from build123d import *

# Parameters (mm, degrees)
SKETCH1_R            = 15
BOSS_EXTRUDE1_DEPTH  = 2.75
SKETCH1_3_W          = 2
SKETCH1_3_H          = 25
BOSS_EXTRUDE2_DEPTH  = 4.25
CUT_EXTRUDE1_DEPTH   = 49.073511417
M4_CLEARANCE_HOLE1_D = 4.5


with BuildPart() as part:
    # Sketch1 → Boss-Extrude1 (new, symmetric)
    with BuildSketch(Plane.XY):
        Polygon((19, 12.5), (21, 12.5), (10, 23), (10, 21), (-10, 21), (-10, 23), (-21, 12.5), (-19, 12.5), (-19, -12.5), (-21, -12.5), (-21, -23), (-17, -23), (-17, -20), (-14, -20), (-14, -23), (-10, -23), (-10, -21), (10, -21), (10, -23), (14, -23), (14, -20), (17, -20), (17, -23), (21, -23), (21, -12.5), (19, -12.5), align=None)
        Circle(SKETCH1_R, mode=Mode.SUBTRACT)
    extrude(amount=BOSS_EXTRUDE1_DEPTH, both=True)

    # Sketch1<3> → Boss-Extrude2 (add, symmetric)
    with BuildSketch(Plane.XY):
        with Locations((-20, 0)):
            Rectangle(SKETCH1_3_W, SKETCH1_3_H)
        with Locations((20, 0)):
            Rectangle(SKETCH1_3_W, SKETCH1_3_H)
    extrude(amount=BOSS_EXTRUDE2_DEPTH, both=True)

    # Sketch2 → Cut-Extrude1 (cut, through all)
    with BuildSketch(Plane.ZY.offset(21)):
        Polygon((4.25, -12.5), (4.25, -8.5), (2.75, -12.5), align=None)
        Polygon((-2.75, -12.5), (-4.25, -8.5), (-4.25, -12.5), align=None)
        Polygon((-4.25, 8.5), (-2.75, 12.5), (-4.25, 12.5), align=None)
        Polygon((4.25, 12.5), (2.75, 12.5), (4.25, 8.5), align=None)
    extrude(amount=-CUT_EXTRUDE1_DEPTH, mode=Mode.SUBTRACT)

    # M4 Clearance Hole1 (through all)
    with Locations(Plane(origin=(0, 21, 0), x_dir=(1, 0, 0), z_dir=(0, 1, 0))):
        with Locations((0, 0)):
            Hole(M4_CLEARANCE_HOLE1_D / 2)


solid = part.part
Work out the finished part from the listing and answer in its coordinate system (mm). A direction names the side the tool comes from. Round coordinates to 2 decimals unless told otherwise and drop trailing zeros. Order: outer loops, then holes, each group sorted by start corner. A loop starts at its lowest first (then second) coordinate and runs counter-clockwise, first axis right, second up. Notation, with made-up numbers: M 62.25,63 L 84.25,63 A17 ccw 84.25,85 Z; hole C -31.75,-21.5 d3. An arc over 180 degrees is marked long. Put each result on its own line as item: value. Start each with the question number.
Q1. Straight lines are drawn through the part: L1, parallel to X at y = -3, z = 4; L2, parallel to Z at x = 0, y = -18.5; L3, parallel to Z at x = -6, y = 17. For each, find the intervals that lie inside material, in ascending order. Write a range as [from, to].
Q2. Section A-A, the plane x = 0 is taken. Write down the section's boundary in (y, z).
Q3. Section B-B, the plane y = 0 is taken. Write down the section's boundary in (x, z), and give its area (3 significant figures).
Q4. Section D-D, the plane x = 9 is taken. Write down the section's boundary in (y, z).
Q5. For a pull along Z with two mould halves and no side action, classify faces 1 (the flat face through (-15.423, 17.824, 0.038)), 2 (the flat face through (-5, -15, -2.75)), 3 (the cylindrical face through (0.29, -17.96, -2.23)) as pulls with the +Z half, pulls with the -Z half, needs draft (parallel to the pull), parting line crosses it, or undercut.
Q6. Flat-ended cylindrical pins translate along their axes: pin 1 (12 mm diameter, centred on x = 9, y = 1.5, fed in from +Z); pin 2 (8 mm diameter, centred on x = 14, y = 3.5, fed in from -Z); pin 3 (3.5 mm diameter, centred on x = 15, z = 0.5, fed in from -Y); pin 4 (3 mm diameter, centred on x = -2.5, z = 2.5, fed in from -Y). Find the tip coordinate at first contact, or state that the pin passes through.
Q7. Section C-C, the plane z = 0 is taken. Write down the section's boundary in (x, y).
Q8. A tool of negligible diameter and unlimited length cuts with its end or side. For faces 4 (the flat face through (10, -22, 0)), 5 (the flat face through (19, 0, -3)), 6 (the flat face through (-21, -5, 0)), 7 (the flat face through (-19, 0, 3)), 8 (the flat face through (12, -23, 0)), from which of +Z, -Z, +X, -X, +Y, -Y can it reach the whole face along a straight path? Write none if from no direction.
Findings below:
1. L1: x = [-21, -19], [19, 21]
1. L2: z = [-2.75, -2.25], [2.25, 2.75]
1. L3: z = [-2.75, 2.75]
2. outline: M -21,-2.75 L -15,-2.75 L -15,-2.25 L -21,-2.25 Z; M -21,2.25 L -15,2.25 L -15,2.75 L -21,2.75 Z; M 15,-2.75 L 21,-2.75 L 21,-2.25 L 15,-2.25 Z; M 15,2.25 L 21,2.25 L 21,2.75 L 15,2.75 Z
3. outline: M -21,-4.25 L -19,-4.25 L -19,-2.75 L -15,-2.75 L -15,2.75 L -19,2.75 L -19,4.25 L -21,4.25 Z; M 15,-2.75 L 19,-2.75 L 19,-4.25 L 21,-4.25 L 21,4.25 L 19,4.25 L 19,2.75 L 15,2.75 Z
3. area: 78.0 mm^2
4. outline: M -21,-2.75 L -12,-2.75 L -12,2.75 L -21,2.75 Z; M 12,-2.75 L 21,-2.75 L 21,2.75 L 12,2.75 Z
5. face 1: needs draft
5. face 2: pulls with the -Z half
5. face 3: undercut
6. pin 1: stops at z = 2.75
6. pin 2: stops at z = -2.75
6. pin 3: stops at y = -23
6. pin 4: stops at y = -21
7. outline: M -21,-23 L -17,-23 L -17,-20 L -14,-20 L -14,-23 L -10,-23 L -10,-21 L -2.25,-21 L -2.25,-14.83 A15 cw -2.25,14.83 L -2.25,21 L -10,21 L -10,23 L -21,12.5 Z; M 2.25,-21 L 10,-21 L 10,-23 L 14,-23 L 14,-20 L 17,-20 L 17,-23 L 21,-23 L 21,12.5 L 10,23 L 10,21 L 2.25,21 L 2.25,14.83 A15 cw 2.25,-14.83 Z
8. face 4: +Z, -Z, -Y
8. face 5: -Z, +Y, -Y
8. face 6: +Z, -Z, -X, +Y, -Y
8. face 7: +Z, +Y, -Y
8. face 8: +Z, -Z, +X, -X, -Y
